from build123d import *

# Parameters (mm, degrees)
SKETCH_1_W          = 43.34
SKETCH_1_H          = 43.34
EXTRUDE_1_DEPTH     = 28.5
CUT_EXTRUDE_1_DEPTH = 25.5
SKETCH_3_R          = 4
SKETCH_3_W          = 7.7
SKETCH_3_H          = 10.5
SKETCH_3_W_2        = 15
SKETCH_3_H_2        = 7.7
SKETCH_3_H_3        = 5
EXTRUDE_2_DEPTH     = 11
SKETCH_4_R          = 1.6
CUT_EXTRUDE_2_DEPTH = 40.867628472


with BuildPart() as part:
    # 스케치1 → 보스-돌출1 (new body)
    with BuildSketch(Plane(origin=(0, 0, 0), x_dir=(1, 0, 0), z_dir=(0, 1, 0))):
        Rectangle(SKETCH_1_W, SKETCH_1_H)
    extrude(amount=EXTRUDE_1_DEPTH)

    # 스케치2 → 컷-돌출1 (cut)
    with BuildSketch(Plane(origin=(0, 28.5, 0), x_dir=(1, 0, 0), z_dir=(0, 1, 0))):
        Polygon((-11.5, 21.67), (-11.5, 5.67), (11.5, 5.67), (11.5, 21.67), (21.67, 21.67), (21.67, -21.67), (-21.67, -21.67), (-21.67, 21.67), align=None)
    extrude(amount=-CUT_EXTRUDE_1_DEPTH, mode=Mode.SUBTRACT)

    # 스케치3 → 보스-돌출2 (add)
    with BuildSketch(Plane(origin=(0, 3, 0), x_dir=(1, 0, 0), z_dir=(0, 1, 0))):
        with Locations(Location((-6.17, -3.67, 0), (0, 0, 90))):
            Circle(SKETCH_3_R)
        with Locations(Location((7.67, -11.17, 0), (0, 0, 90))):
            Circle(SKETCH_3_R)
        with Locations((-16.82, -6.92)):
            Rectangle(SKETCH_3_W, SKETCH_3_H)
        with Locations((-7.97, -16.82)):
            Rectangle(SKETCH_3_W_2, SKETCH_3_H_2)
        with Locations((8.03, -18.17)):
            Rectangle(SKETCH_3_W_2, SKETCH_3_H_3)
        with Locations((16.82, -7.42)):
            Rectangle(SKETCH_3_W, SKETCH_3_H)
    extrude(amount=EXTRUDE_2_DEPTH)

    # 스케치4 → 컷-돌출2 (cut, through all)
    with BuildSketch(Plane(origin=(0, 3, 0), x_dir=(1, 0, 0), z_dir=(0, 1, 0))):
        with Locations(Location((-18.67, 18.67, 0), (0, 0, 270))):
            Circle(SKETCH_4_R)
        with Locations(Location((18.67, 18.67, 0), (0, 0, 270))):
            Circle(SKETCH_4_R)
        with Locations(Location((18.67, -18.67, 0), (0, 0, 270))):
            Circle(SKETCH_4_R)
        with Locations(Location((-18.67, -18.67, 0), (0, 0, 270))):
            Circle(SKETCH_4_R)
    extrude(amount=-CUT_EXTRUDE_2_DEPTH, mode=Mode.SUBTRACT)


solid = part.part
For this review, take the finished solid that the model builds, in its own axes (mm). A direction names the side the tool comes from. Round coordinates to 2 decimals unless told otherwise and drop trailing zeros. Order: outer loops, then holes, each group sorted by start corner. A loop starts at its lowest first (then second) coordinate and runs counter-clockwise, first axis right, second up. Notation, with made-up numbers: M -28,60 L 12,60 A21 ccw 12,81 Z; hole C 23.5,-40 d8. An arc over 180 degrees is marked long. Write each question's results on one line, items separated by ' | '. Start each with the question number.
1. Clearance check with flat-ended pins moving along their axes: pin 1 Ø9 at (x, z) = (-6.5, 2.5) entering from +Y; pin 2 Ø4 at (x, z) = (18.67, 18.67) entering from +Y; pin 3 Ø2.5 at (x, z) = (-18.67, -18.67) entering from -Y (3 decimals); pin 4 Ø4 at (x, y) = (15.5, 8) entering from +Z. State where each tip first meets the part, or that it passes through.
2. To check wall thickness, follow L1, parallel to X at y = 1.25, z = -18.67; L2, parallel to Z at x = 6, y = 6.75; L3, parallel to Y at x = 14, z = 5. State the ranges of each line that lie inside material, in increasing order. Write a range as [from, to].
3. Tool access review of faces 4 (the face through (8, 14, 11)), 5 (the face through (6.469, 8.423, 7.355)), 6 (the face through (15.53, 8, 18)): name each direction out of +Z, -Z, +X, -X, +Y, -Y from which nothing blocks a thin tool from reaching the whole face with its end or side.
4. Add section A-A (z = -18.67). State the section outline as (x, y) points, then the cut area to 3 significant figures.
5. Draft analysis for pull direction X (two halves, no side actions). For faces 1 (the face through (-15.47, 8, 17)), 2 (the face through (8, 14, 18)), 3 (the face through (-19.64, 1.52, -19.94)), state which applies: pulls with the +X half, pulls with the -X half, needs draft (parallel to the pull), parting line crosses it, or undercut.
6. Add section D-D (z = -13.5). State the section outline as (x, y) points.
7. Add section B-B (x = 18.67). State the section outline as (y, z) points.
8. Add section C-C (y = 10.25). State the section outline as (x, z) points.
Output values:
1) pin 1: y = 14 | pin 2: y = 3 | pin 3: through | pin 4: z = 20.67
2) L1: [-21.67, -20.27], [-17.07, 17.07], [20.27, 21.67] | L2: [-21.67, -5.67], [7.54, 14.8], [15.67, 20.67] | L3: [0, 14]
3) face 4: +Z, +X, -X, +Y | face 5: +Y | face 6: +Z, +X, +Y
4) outline: M -21.67,0 L -20.27,0 L -20.27,3 L -21.67,3 Z; M -17.07,0 L 17.07,0 L 17.07,3 L 11.5,3 L 11.5,28.5 L -11.5,28.5 L -11.5,3 L -17.07,3 Z; M 20.27,0 L 21.67,0 L 21.67,3 L 20.27,3 Z | area: 697 mm^2
5) face 1: pulls with the -X half | face 2: needs draft | face 3: undercut
6) outline: M -21.67,0 L 21.67,0 L 21.67,3 L 11.5,3 L 11.5,28.5 L -11.5,28.5 L -11.5,3 L -21.67,3 Z
7) outline: M 0,-21.67 L 3,-21.67 L 3,-20.27 L 0,-20.27 Z; M 0,-17.07 L 3,-17.07 L 3,2.17 L 14,2.17 L 14,12.67 L 3,12.67 L 3,17.07 L 0,17.07 Z; M 0,20.27 L 3,20.27 L 3,21.67 L 0,21.67 Z
8) outline: M -20.67,1.67 L -12.97,1.67 L -12.97,12.17 L -20.67,12.17 Z; M -15.47,12.97 L -0.47,12.97 L -0.47,20.67 L -15.47,20.67 Z; M -11.5,-21.67 L 11.5,-21.67 L 11.5,-5.67 L -11.5,-5.67 Z; C -6.17,3.67 d8; M 0.53,15.67 L 15.53,15.67 L 15.53,20.67 L 0.53,20.67 Z; C 7.67,11.17 d8; M 12.97,2.17 L 20.67,2.17 L 20.67,12.67 L 12.97,12.67 Z
